The drawing under review shows one solid part. Ordinate dimensions are in mm from its lowest x, y, z. Coordinates: 2 decimals unless noted, no trailing zeros. Order: outer loops, then holes, each group sorted by start corner. A loop starts at its lowest first (then second) coordinate and runs counter-clockwise, first axis right, second up.
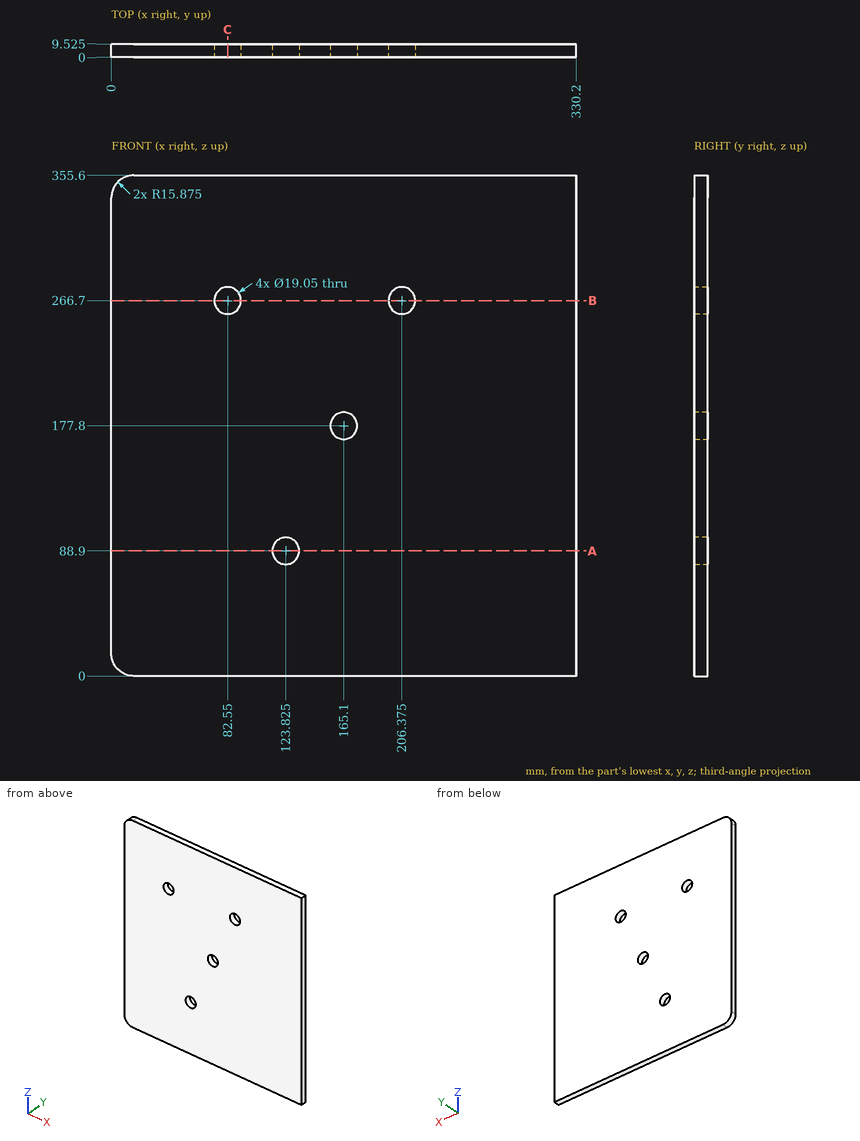
1. To check wall thickness, follow line 1 (X direction, y = 5.75, z = 266.7) (3 decimals); line 2 (X direction, y = 3.75, z = 88.9); line 3 (X direction, y = 2, z = 177.8) (3 decimals). State the ranges of each line that lie inside material, in increasing order.
2. Add section C-C (x = 82.55). Give the boundary of the cut face in (y, z) (3 decimals).
3. Add section A-A (z = 88.9). Give the boundary of the cut face in (x, y) (3 decimals).
4. Insertion check: pin 1 (22 mm diameter, centred on x = 206.375, z = 266.7, fed in from +Y) (3 decimals). The pin has a flat end and moves straight along its axis. Give the tip position at first contact, or say it passes through.
5. Add section B-B (z = 266.7). Give the boundary of the cut face in (x, y) (3 decimals), and give its area (3 significant figures).
Solution:
1. line 1: x = 0 to 73.025, 92.075 to 196.85, 215.9 to 330.2
1. line 2: x = 0 to 114.3, 133.35 to 330.2
1. line 3: x = 0 to 155.575, 174.625 to 330.2
2. outline: (0, 0) - (9.525, 0) - (9.525, 257.175) - (0, 257.175) - close; (0, 276.225) - (9.525, 276.225) - (9.525, 355.6) - (0, 355.6) - close
3. outline: (0, 0) - (114.3, 0) - (114.3, 9.525) - (0, 9.525) - close; (133.35, 0) - (330.2, 0) - (330.2, 9.525) - (133.35, 9.525) - close
4. pin 1: stops at y = 9.525
5. outline: (0, 0) - (73.025, 0) - (73.025, 9.525) - (0, 9.525) - close; (92.075, 0) - (196.85, 0) - (196.85, 9.525) - (92.075, 9.525) - close; (215.9, 0) - (330.2, 0) - (330.2, 9.525) - (215.9, 9.525) - close
5. area: 2,780 mm2
